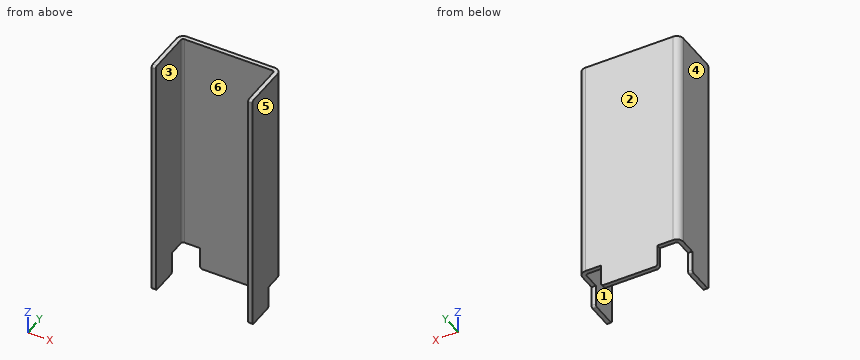
```python
from build123d import *

# Parameters (mm, degrees)
F1_DEPTH = 50
F2_W     = 25
F2_H     = 20
F3_DEPTH = 1.9
F4_W     = 12.5
F4_H     = 10
F5_DEPTH = 1.9
F7_R     = 1


with BuildPart() as f1:
    # F0 (on Top) → F1 (new body, symmetric)
    with BuildSketch(Plane.XY):
        with BuildLine():
            Line((-19.5, 10.25), (19.5, 10.25))
            ThreePointArc((19.5, 10.25), (20.2071067812, 9.9571067812), (20.5, 9.25))
            Line((20.5, 9.25), (20.5, -10.25))
            Line((20.5, -10.25), (22.4, -10.25))
            Line((22.4, -10.25), (22.4, 9.25))
            ThreePointArc((22.4, 9.25), (21.5506096654, 11.3006096654), (19.5, 12.15))
            Line((19.5, 12.15), (-19.5, 12.15))
            ThreePointArc((-19.5, 12.15), (-21.5506096654, 11.3006096654), (-22.4, 9.25))
            Line((-22.4, 9.25), (-22.4, -10.25))
            Line((-22.4, -10.25), (-20.5, -10.25))
            Line((-20.5, -10.25), (-20.5, 9.25))
            ThreePointArc((-20.5, 9.25), (-20.2071067812, 9.9571067812), (-19.5, 10.25))
        make_face()
    extrude(amount=F1_DEPTH, both=True)

    # F2 (on face) → F3 (join, through all)
    with BuildSketch(Plane(origin=(0, 12.15, 0), x_dir=(-1, 0, 0), z_dir=(0, 1, 0))):
        with Locations((0, -50)):
            Rectangle(F2_W, F2_H)
    extrude(amount=-F3_DEPTH)

    # F4 (on face) → F5 (join, through all)
    with BuildSketch(Plane.YZ.offset(22.4)):
        with Locations((-4, -55)):
            Rectangle(F4_W, F4_H)
    extrude(amount=-F5_DEPTH)

    # F6: F1 across plane


with BuildPart() as f1_1:
    add(f1.part)
    add(f1.part.mirror(Plane.YZ))

    # F7
    f7_edges = [f1_1.edges().sort_by_distance(p)[0] for p in [
        (21.45, -10.25, 50),
        (-21.45, -10.25, 50),
        (12.5, 11.2, -60),
        (-12.5, 11.2, -60),
        (21.45, 2.25, -60),
        (-21.45, 2.25, -60),
        (21.45, -10.25, -60),
        (-21.45, -10.25, -60),
    ]]
    fillet(f7_edges, radius=F7_R)


solid = f1_1.part
```
Source: CAD feature listing. Evaluate the final solid. Frame: model axes, mm. Face numbers are marked on the shaded views. A direction names the side the tool comes from. Coordinates: 2 decimals unless noted, no trailing zeros. Loops run counter-clockwise (first coordinate to the right, second up) from the corner with the lowest first, then second, coordinate; pieces in that order, holes last. Notation, with made-up numbers: M 47,77.25 L 74,77.25 A17 ccw 74,89.25 Z; hole C 6,74 d5. An arc over 180 degrees is marked long. Use CSV: the item, a comma, the result in double quotes.
(1) Cut plane B-B on z = -5. Return loops of the section in (x, y), and give its area (3 significant figures).
Answers follow:
outline,"M -22.4,-10.25 L -20.5,-10.25 L -20.5,9.25 A1 cw -19.5,10.25 L 19.5,10.25 A1 cw 20.5,9.25 L 20.5,-10.25 L 22.4,-10.25 L 22.4,9.25 A2.9 ccw 19.5,12.15 L -19.5,12.15 A2.9 ccw -22.4,9.25 Z"
area,"160 mm²"
(2) Cut plane A-A on y = -1.25. Return loops of the section in (x, z).
Answers follow:
outline,"M -22.4,-60 L -20.5,-60 L -20.5,50 L -22.4,50 Z; M 20.5,-60 L 22.4,-60 L 22.4,50 L 20.5,50 Z"
(3) Line query: line 1 (X direction, y = -0.25, z = 22); line 2 (Y direction, x = -19.5, z = 35). Output: solid intervals per line, ascending. Write a range as [from, to].
Answers follow:
line 1,"[-22.4, -20.5], [20.5, 22.4]"
line 2,"[10.25, 12.15]"
(4) Contact query for flat-ended pins moving along their axis: pin 1 (8 mm diameter, centred on x = -15, y = 7.5, fed in from -Z); pin 2 (1.5 mm diameter, centred on y = 11, z = -53, fed in from -X); pin 3 (1 mm diameter, centred on y = 11.5, z = -56.5, fed in from +X). Output: stop coordinate, or through.
Answers follow:
pin 1,"z = -59.8"
pin 2,"x = -12.5"
pin 3,"x = 12.5"
(5) Reachability of the marked faces 5 and 6 from +Z, -Z, +X, -X, +Y, -Y: full face, straight path, thin tool, end or side. Return the list, or none.
Answers follow:
face 5,"+Z, -Z, +X, +Y, -Y"
face 6,"+Z, -Z, -Y"
(6) Cut plane C-C on y = 5.75. Return loops of the section in (x, z), and give its area (3 significant figures).
Answers follow:
outline,"M -22.4,-50 L -20.5,-50 L -20.5,50 L -22.4,50 Z; M 20.5,-50 L 22.4,-50 L 22.4,50 L 20.5,50 Z"
area,"380 mm²"
(7) Draft query along X for the marked faces 1, 2, 3 and 4. Return one class per face: pulls with the +X half, pulls with the -X half, needs draft (parallel to the pull), parting line crosses it, or undercut.
Answers follow:
face 1,"undercut"
face 2,"needs draft"
face 3,"undercut"
face 4,"pulls with the -X half"
(8) Cut plane D-D on x = 14.5. Return loops of the section in (y, z).
Answers follow:
outline,"M 10.25,-50 L 12.15,-50 L 12.15,50 L 10.25,50 Z"
